Source: CAD feature listing. Evaluate the final solid. Frame: model axes, mm. A direction names the side the tool comes from. Round coordinates to 2 decimals unless told otherwise and drop trailing zeros. Write each loop counter-clockwise with the first axis right and the second up, starting at its lowest first coordinate (ties: lowest second). Pieces come first, ordered by that corner, then holes. Notation, with made-up numbers: M -25,-8.5 L 8,-8.5 A23 cw 8,16.5 Z; hole C -40,32.5 d4. An arc over 180 degrees is marked long. Answer in a Markdown table with one row per item.
Autodesk Inventor part; units mm, degrees
ref_plane "YZ Plane" through (0, 0, 0) normal (1, 0, 0) x (0, 1, 0)
ref_plane "XZ Plane" through (0, 0, 0) normal (0, 1, 0) x (-1, 0, 0)
ref_plane "XY Plane" through (0, 0, 0) normal (0, 0, 1) x (1, 0, 0)
sketch "Sketch1" plane through (0, 0, 0) normal (1, 0, 0) x (0, 1, 0)
  line L0 (-32.6, 45) -> (32.6, 45)
  line L1 (32.6, 45) -> (32.6, -45)
  line L2 (32.6, -45) -> (-32.6, -45)
  line L3 (-32.6, -45) -> (-32.6, 45)
  line L4 (-32.6, 45) -> (32.6, -45) construction
  line L5 (32.6, 45) -> (-32.6, -45) construction
  point P0 (0, 0)
  dimension "d0" = 65.2
  dimension "d1" = 90
extrude "Extrusion1" add sketch "Sketch1" along normal blind 10
sketch "Sketch2" plane through (0, 32.6, 45) normal (0, 1, 0) x (1, 0, 0)
  line L0 (0, 0) -> (10, 0)
  line L1 (0, 0) -> (5, 0)
  line L2 (5, 0) -> (5, 20)
  circle A0 centre (5, 20) radius 2
  line L3 (0, 45) -> (10, 45)
  line L4 (0, 90) -> (10, 90)
  line L5 (0, 90) -> (5, 90)
  line L6 (5, 90) -> (5, 70)
  circle A1 centre (5, 70) radius 2
  dimension "d4" = 5
  dimension "d5" = 20
  dimension "d6" = 4
extrude "Extrusion2" cut sketch "Sketch2" against normal blind 25
thread "Thread1"
thread "Thread2"
sketch "Sketch3" plane through (0, -32.6, -45) normal (0, -1, 0) x (1, 0, 0)
  line L0 (0, 45) -> (9.9068, 45)
  line L1 (10, 0) -> (10, 90)
  line L2 (10, 90) -> (5, 90)
  line L3 (0, 90) -> (10, 90)
  line L4 (5, 90) -> (5, 70)
  circle A0 centre (5, 70) radius 2
  line L5 (10, 0) -> (5, 0)
  line L6 (0, 0) -> (10, 0)
  line L7 (5, 0) -> (5, 20)
  circle A1 centre (5, 20) radius 2
  dimension "d13" = 5
  dimension "d14" = 20
  dimension "d15" = 4
extrude "Extrusion3" cut sketch "Sketch3" against normal blind 25
thread "Thread3"
thread "Thread4"
sketch "Sketch6" plane through (10, 0, 0) normal (1, 0, 0) x (0, 0, -1)
  line L0 (-45, -32.6) -> (45, -32.6)
  line L1 (0, -32.6) -> (0, 1.6)
  line L2 (-12.5, -7.9) -> (12.5, -7.9)
  line L3 (12.5, -7.9) -> (12.5, 11.1)
  line L4 (12.5, 11.1) -> (-12.5, 11.1)
  line L5 (-12.5, 11.1) -> (-12.5, -7.9)
  line L6 (-12.5, -7.9) -> (12.5, 11.1) construction
  line L7 (12.5, -7.9) -> (-12.5, 11.1) construction
  line L8 (45, 32.6) -> (-45, 32.6)
  point P0 (0, 0)
  dimension "d29" = 34.2
  dimension "d30" = 25
  dimension "d31" = 19
extrude "Extrusion6" cut sketch "Sketch6" against normal blind 10
sketch "Sketch10" plane through (10, 0, 0) normal (1, 0, 0) x (0, 0, -1)
  circle A0 centre (-27.5, 25.1) radius 2.5
sketch "Sketch11" plane through (0, 0, 0) normal (-1, 0, 0) x (0, 0, 1)
  circle A0 centre (27.5, 25.1) radius 2.5
sketch "Sketch12" plane through (0, -32.6, 45) normal (0, 0, 1) x (1, 0, 0)
  line L0 (0, 65.2173) -> (5, 65.2173)
  line L1 (5, 65.2173) -> (5, 60.2173)
  line L2 (0, 32.6) -> (10, 32.6)
  line L3 (10, 0) -> (10, 65.2)
  circle A0 centre (5, 60.2173) radius 2
  circle A1 centre (5, 4.9827) radius 2
  dimension "d46" = 5
  dimension "d47" = 5
  dimension "d48" = 4
extrude "Extrusion9" cut sketch "Sketch12" against normal blind 15
sketch "Sketch13" plane through (10, 0, 0) normal (1, 0, 0) x (0, 0, -1)
  point P0 (0, 0)
sketch "Sketch14" plane through (0, -32.6, -45) normal (0, 0, -1) x (-1, 0, 0)
  line L0 (0, 65.2) -> (-10, 65.2)
  line L1 (-10, 65.2) -> (-5, 65.2)
  line L2 (-5, 65.2) -> (-5, 60.2)
  circle A0 centre (-5, 60.2) radius 2
  line L3 (0, 32.6) -> (-10, 32.6)
  line L4 (-10, 43.7) -> (-10, 24.7)
  circle A1 centre (-5, 5) radius 2
  dimension "d51" = 5
  dimension "d52" = 5
  dimension "d53" = 4
extrude "Extrusion10" cut sketch "Sketch14" against normal blind 15
thread "Thread5"
thread "Thread6"
thread "Thread7"
thread "Thread8"
properties part number "Rb PEEK - Largo"
Q1. Pull-direction query (Y, two-part tool) for faces 1 (the flat face through (5, 11.1, 0)), 2 (the flat face through (5, -7.6, -25)), 3 (the flat face through (0, 14, 1)); classes: pulls with the +Y half, pulls with the -Y half, needs draft (parallel to the pull), parting line crosses it, or undercut.
Solutions:
| item | result |
|---|---|
| face 1 | undercut |
| face 2 | pulls with the -Y half |
| face 3 | needs draft |
Q2. Section B-B (x = 2). Return loops of the section in (y, z), and give its area (3 significant figures).
Solutions:
| item | result |
|---|---|
| outline | M -32.6,-45 L 32.6,-45 L 32.6,45 L -32.6,45 Z; hole M -7.9,-12.5 L 11.1,-12.5 L 11.1,12.5 L -7.9,12.5 Z |
| area | 5,390 mm2 |
Q3. Section A-A (z = -8.5). Return loops of the section in (x, y).
Solutions:
| item | result |
|---|---|
| outline | M 0,-32.6 L 10,-32.6 L 10,-7.9 L 0,-7.9 Z; M 0,11.1 L 10,11.1 L 10,32.6 L 0,32.6 Z |
Q4. Section D-D (z = 25). Return loops of the section in (x, y).
Solutions:
| item | result |
|---|---|
| outline | M 0,-32.6 L 3,-32.6 L 3,-7.6 L 7,-7.6 L 7,-32.6 L 10,-32.6 L 10,32.6 L 7,32.6 L 7,7.6 L 3,7.6 L 3,32.6 L 0,32.6 Z |
Q5. Access query for faces 4 (the flat face through (5, 2, 12.5)), 5 (the flat face through (5, -28, 30)), 6 (the cylindrical face through (5.26, 29.583, -37.605)). Directions: +Z, -Z, +X, -X, +Y, -Y. A direction counts if a zero-diameter tool reaches every point of the face in a straight line with its end or side. Return the directions, or none.
Solutions:
| item | result |
|---|---|
| face 4 | +X, -X |
| face 5 | +Z |
| face 6 | -Z |
Q6. Material intervals for probe 1 along Y at (x, z) = (5, 36.5); probe 2 along Z at (x, y) = (5, 23.75); probe 3 along Z at (x, y) = (3.5, -4), sorted ascending.
Solutions:
| item | result |
|---|---|
| probe 1 | y = -32.6 to -29.62, -25.62 to 25.62, 29.62 to 32.6 |
| probe 2 | z = -45 to -27, -23 to 23, 27 to 45 |
| probe 3 | z = -45 to -12.5, 12.5 to 45 |
Q7. Section C-C (y = 23). Return loops of the section in (x, z), and give its area (3 significant figures).
Solutions:
| item | result |
|---|---|
| outline | M 0,-45 L 10,-45 L 10,45 L 0,45 Z; hole C 5,-25 d4; hole C 5,25 d4 |
| area | 875 mm2 |
Q8. Contact query for flat-ended pins moving along their axis: pin 1 Ø2 at (y, z) = (-21, -18.5) entering from -X; pin 2 Ø2.5 at (x, y) = (5, 27.62) entering from -Z; pin 3 Ø3.5 at (x, y) = (5, 27.6) entering from +Z. Output: stop coordinate, or through.
Solutions:
| item | result |
|---|---|
| pin 1 | stops at x = 0 |
| pin 2 | stops at z = -30 |
| pin 3 | stops at z = 30 |
